```python
from build123d import *

# Parameters (mm, degrees)
BOSS_EXTRUDE1_DEPTH      = 6.35
BOSS_EXTRUDE1_DEPTH_BACK = 6.35
SKETCH2_R                = 25.4
SHELL1_T                 = -2
BOSS_EXTRUDE2_DEPTH      = 6.35
BOSS_EXTRUDE2_DEPTH_BACK = 6.35
CUT_EXTRUDE1_DEPTH       = 44.444866103
SKETCH10_W               = 3.18
SKETCH10_H               = 12.7
CUT_EXTRUDE2_DEPTH       = 44.444866103
FILLET1_R                = 3.175
CUT_EXTRUDE4_REACH       = 63.003
SKETCH11_W               = 12.7
SKETCH11_H               = 3.18
FILLET2_R                = 1.5875
FILL_START               = -6.35
FILL_PATTERN1_OUTLINE_R  = 1.190625
FILL_PATTERN1_DEPTH      = 2


# Read off the part's stored shape, not the designer's step: Fill Pattern1
with BuildPart() as part:
    # Sketch2 → Boss-Extrude1 (new, two sides: drawn at the far end of the back side and taken through both)
    with BuildSketch(Plane(origin=(0, 0, 0), x_dir=(1, 0, 0), z_dir=(0, 1, 0)).offset(-BOSS_EXTRUDE1_DEPTH_BACK)):
        with Locations(Location((0, 0, 0), (0, 0, 270))):
            Circle(SKETCH2_R)
    extrude(amount=BOSS_EXTRUDE1_DEPTH + BOSS_EXTRUDE1_DEPTH_BACK)

    # Shell1
    shell1_openings = [part.faces().sort_by_distance(p)[0] for p in [
        (0, 6.35, 0),
    ]]
    offset(amount=SHELL1_T, openings=shell1_openings, kind=Kind.INTERSECTION)

    # Sketch7 → Boss-Extrude2 (add, two sides: drawn at the far end of the back side and taken through both)
    with BuildSketch(Plane(origin=(0, 0, 0), x_dir=(1, 0, 0), z_dir=(0, 1, 0)).offset(-BOSS_EXTRUDE2_DEPTH_BACK)):
        with BuildLine():
            Line((23.348661632, 10), (32.878661632, 10))
            Line((32.878661632, 10), (32.878661632, -10))
            Line((32.878661632, -10), (23.348661632, -10))
            ThreePointArc((23.348661632, -10), (25.4, 0), (23.348661632, 10))
        make_face()
    extrude(amount=BOSS_EXTRUDE2_DEPTH + BOSS_EXTRUDE2_DEPTH_BACK)

    # Sketch9 → Cut-Extrude1 (cut, through all)
    with BuildSketch(Plane(origin=(0, 6.35, 0), x_dir=(1, 0, 0), z_dir=(0, 1, 0))):
        with BuildLine():
            Line((26.003661632, 7.5), (27.053661632, 7.5))
            ThreePointArc((27.053661632, 7.5), (27.760768413, 7.207106781), (28.053661632, 6.5))
            Line((28.053661632, 6.5), (28.053661632, -6.5))
            ThreePointArc((28.053661632, -6.5), (27.760768413, -7.207106781), (27.053661632, -7.5))
            Line((27.053661632, -7.5), (26.003661632, -7.5))
            ThreePointArc((26.003661632, -7.5), (25.296554851, -7.207106781), (25.003661632, -6.5))
            Line((25.003661632, -6.5), (25.003661632, 6.5))
            ThreePointArc((25.003661632, 6.5), (25.296554851, 7.207106781), (26.003661632, 7.5))
        make_face()
    extrude(amount=-CUT_EXTRUDE1_DEPTH, mode=Mode.SUBTRACT)

    # Sketch10 → Cut-Extrude2 (cut, through all)
    with BuildSketch(Plane(origin=(0, 6.35, 0), x_dir=(1, 0, 0), z_dir=(0, 1, 0))):
        with Locations((31.288661632, 0)):
            Rectangle(SKETCH10_W, SKETCH10_H)
    extrude(amount=-CUT_EXTRUDE2_DEPTH, mode=Mode.SUBTRACT)

    # Fillet1
    fillet1_edges = [part.edges().sort_by_distance(p)[0] for p in [
        (23.348661632, 0, 10),
        (23.348661632, 0, -10),
        (32.878661632, 0, -10),
        (32.878661632, 0, 10),
    ]]
    fillet(fillet1_edges, radius=FILLET1_R)

    # Sketch11 → Cut-Extrude4 (cut, up to next)
    with BuildSketch(Plane(origin=(29.698661632, 0, 0), x_dir=(0, 0, -1), z_dir=(1, 0, 0)), mode=Mode.PRIVATE) as cut_extrude4_sk1:
        with Locations((0, -4.76)):
            Rectangle(SKETCH11_W, SKETCH11_H)
    cut_extrude4_tool1 = extrude(cut_extrude4_sk1.sketch, amount=-CUT_EXTRUDE4_REACH, mode=Mode.PRIVATE) & part.part
    add(cut_extrude4_tool1.solids().sort_by_distance((29.698662, -4.76, 0))[0], mode=Mode.SUBTRACT)

    # Fillet2
    fillet2_edges = [part.edges().sort_by_distance(p)[0] for p in [
        (29.698661632, 1.59, -6.35),
        (29.698661632, 1.59, 6.35),
    ]]
    fillet(fillet2_edges, radius=FILLET2_R)

    # Fill Pattern1 outline → Fill Pattern1 (cut)
    with BuildSketch(Plane(origin=(0, 0, 0), x_dir=(1, 0, 0), z_dir=(0, 1, 0)).offset(FILL_START)):
        with Locations((0, -19.999996628)):
            Circle(FILL_PATTERN1_OUTLINE_R)
        with Locations((4.330127019, -12.499996628)):
            Circle(FILL_PATTERN1_OUTLINE_R)
        with Locations((4.330127019, -7.499996628)):
            Circle(FILL_PATTERN1_OUTLINE_R)
        with Locations((8.660254038, -4.999996628)):
            Circle(FILL_PATTERN1_OUTLINE_R)
        with Locations((8.660254038, 3.372e-06)):
            Circle(FILL_PATTERN1_OUTLINE_R)
        with Locations((12.990381057, 2.500003372)):
            Circle(FILL_PATTERN1_OUTLINE_R)
        with Locations((12.990381057, 7.500003372)):
            Circle(FILL_PATTERN1_OUTLINE_R)
        with Locations((8.660254038, 15.000003372)):
            Circle(FILL_PATTERN1_OUTLINE_R)
        with Locations((-12.990381057, -12.499996628)):
            Circle(FILL_PATTERN1_OUTLINE_R)
        with Locations((-4.330127019, -12.499996628)):
            Circle(FILL_PATTERN1_OUTLINE_R)
        with Locations((0, -9.999996628)):
            Circle(FILL_PATTERN1_OUTLINE_R)
        with Locations((0, -4.999996628)):
            Circle(FILL_PATTERN1_OUTLINE_R)
        with Locations((4.330127019, -2.499996628)):
            Circle(FILL_PATTERN1_OUTLINE_R)
        with Locations((4.330127019, 2.500003372)):
            Circle(FILL_PATTERN1_OUTLINE_R)
        with Locations((8.660254038, 5.000003372)):
            Circle(FILL_PATTERN1_OUTLINE_R)
        with Locations((8.660254038, 10.000003372)):
            Circle(FILL_PATTERN1_OUTLINE_R)
        with Locations((17.320508076, 10.000003372)):
            Circle(FILL_PATTERN1_OUTLINE_R)
        with Locations((-4.330127019, -17.499996628)):
            Circle(FILL_PATTERN1_OUTLINE_R)
        with Locations((4.330127019, -17.499996628)):
            Circle(FILL_PATTERN1_OUTLINE_R)
        with Locations((8.660254038, -14.999996628)):
            Circle(FILL_PATTERN1_OUTLINE_R)
        with Locations((17.320508076, -4.999996628)):
            Circle(FILL_PATTERN1_OUTLINE_R)
        with Locations((17.320508076, -9.999996628)):
            Circle(FILL_PATTERN1_OUTLINE_R)
        with Locations((12.990381057, -12.499996628)):
            Circle(FILL_PATTERN1_OUTLINE_R)
        with Locations((0, -14.999996628)):
            Circle(FILL_PATTERN1_OUTLINE_R)
        with Locations((-8.660254038, -14.999996628)):
            Circle(FILL_PATTERN1_OUTLINE_R)
        with Locations((12.990381057, 12.500003372)):
            Circle(FILL_PATTERN1_OUTLINE_R)
        with Locations((17.320508076, 5.000003372)):
            Circle(FILL_PATTERN1_OUTLINE_R)
        with Locations((17.320508076, 3.372e-06)):
            Circle(FILL_PATTERN1_OUTLINE_R)
        with Locations((12.990381057, -2.499996628)):
            Circle(FILL_PATTERN1_OUTLINE_R)
        with Locations((12.990381057, -7.499996628)):
            Circle(FILL_PATTERN1_OUTLINE_R)
        with Locations((8.660254038, -9.999996628)):
            Circle(FILL_PATTERN1_OUTLINE_R)
        with Locations((-8.660254038, 10.000003372)):
            Circle(FILL_PATTERN1_OUTLINE_R)
        with Locations((-8.660254038, 5.000003372)):
            Circle(FILL_PATTERN1_OUTLINE_R)
        with Locations((-12.990381057, 2.500003372)):
            Circle(FILL_PATTERN1_OUTLINE_R)
        with Locations((-12.990381057, -2.499996628)):
            Circle(FILL_PATTERN1_OUTLINE_R)
        with Locations((0, 10.000003372)):
            Circle(FILL_PATTERN1_OUTLINE_R)
        with Locations((0, 15.000003372)):
            Circle(FILL_PATTERN1_OUTLINE_R)
        with Locations((-17.320508076, -4.999996628)):
            Circle(FILL_PATTERN1_OUTLINE_R)
        with Locations((-12.990381057, 7.500003372)):
            Circle(FILL_PATTERN1_OUTLINE_R)
        with Locations((-12.990381057, 12.500003372)):
            Circle(FILL_PATTERN1_OUTLINE_R)
        with Locations((-8.660254038, 15.000003372)):
            Circle(FILL_PATTERN1_OUTLINE_R)
        with Locations((-17.320508076, 10.000003372)):
            Circle(FILL_PATTERN1_OUTLINE_R)
        with Locations((-17.320508076, 5.000003372)):
            Circle(FILL_PATTERN1_OUTLINE_R)
        with Locations((-17.320508076, 3.372e-06)):
            Circle(FILL_PATTERN1_OUTLINE_R)
        with Locations((-4.330127019, 17.500003372)):
            Circle(FILL_PATTERN1_OUTLINE_R)
        with Locations((-4.330127019, 12.500003372)):
            Circle(FILL_PATTERN1_OUTLINE_R)
        with Locations((0, 5.000003372)):
            Circle(FILL_PATTERN1_OUTLINE_R)
        with Locations((0, 3.372e-06)):
            Circle(FILL_PATTERN1_OUTLINE_R)
        with Locations((-4.330127019, -2.499996628)):
            Circle(FILL_PATTERN1_OUTLINE_R)
        with Locations((-4.330127019, -7.499996628)):
            Circle(FILL_PATTERN1_OUTLINE_R)
        with Locations((-8.660254038, -9.999996628)):
            Circle(FILL_PATTERN1_OUTLINE_R)
        with Locations((-17.320508076, -9.999996628)):
            Circle(FILL_PATTERN1_OUTLINE_R)
        with Locations((4.330127019, 17.500003372)):
            Circle(FILL_PATTERN1_OUTLINE_R)
        with Locations((-4.330127019, 7.500003372)):
            Circle(FILL_PATTERN1_OUTLINE_R)
        with Locations((-4.330127019, 2.500003372)):
            Circle(FILL_PATTERN1_OUTLINE_R)
        with Locations((-8.660254038, 3.372e-06)):
            Circle(FILL_PATTERN1_OUTLINE_R)
        with Locations((-8.660254038, -4.999996628)):
            Circle(FILL_PATTERN1_OUTLINE_R)
        with Locations((-12.990381057, -7.499996628)):
            Circle(FILL_PATTERN1_OUTLINE_R)
        with Locations((0, 20.000003372)):
            Circle(FILL_PATTERN1_OUTLINE_R)
        with Locations((4.330127019, 12.500003372)):
            Circle(FILL_PATTERN1_OUTLINE_R)
        with Locations((4.330127019, 7.500003372)):
            Circle(FILL_PATTERN1_OUTLINE_R)
    extrude(amount=FILL_PATTERN1_DEPTH, mode=Mode.SUBTRACT)


solid = part.part
```
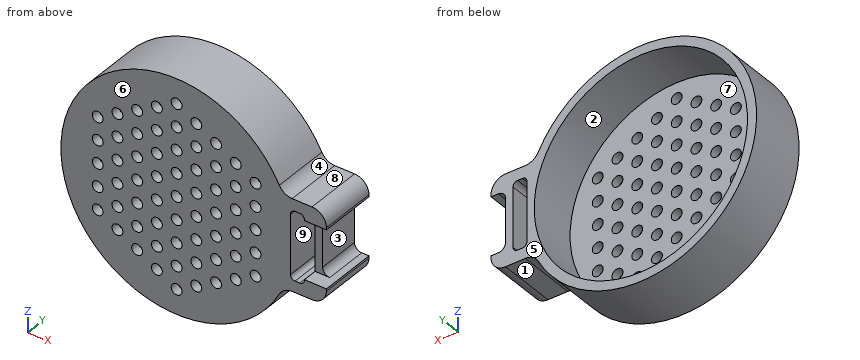
For this review, take the finished solid that the model builds, in its own axes (mm). Face numbers are marked on the shaded views. A direction names the side the tool comes from. Round coordinates to 2 decimals unless told otherwise and drop trailing zeros. Use one line per item in the form item = value.
Q1. Consider section A-A (y = 4). State how many separate pieces and enclosed holes the cut face has, then the cut area to 3 significant figures.
Resolved:
separate_pieces = 1
enclosed_holes = 2
area = 382 mm²
Q2. To check wall thickness, follow probe 1 along Z at (x, y) = (26.5, 4.25); probe 2 along Z at (x, y) = (0.5, -4.25); probe 3 along X at (y, z) = (-5.5, -18). State the ranges of each line that lie inside material, in increasing order. Write a range as from..to.
Resolved:
probe_1 = -10..-7.5, 7.5..10
probe_2 = -25.4..-23.39, 23.39..25.4
probe_3 = -17.92..-5.41, -3.25..3.25, 5.41..17.92
Q3. Machinability: for the marked faces 5, 6, 7, 8 and 9, which of the approach directions +Z, -Z, +X, -X, +Y, -Y give a long, thin tool a straight path to every point of the face, cutting with its end or side? Answer none if there is none.
Resolved:
face_5 = +Z, -Z, +X, -X, +Y
face_6 = +Z, -Z, +X, -X, -Y
face_7 = +Y
face_8 = +Z, +X, +Y, -Y
face_9 = +Y, -Y
Q4. The part is to be moulded in two halves that separate along Z. For the marked faces 1, 2, 3 and 4, say which applies: released by +Z, released by -Z, zero draft, split by the parting line, or undercut.
Resolved:
face_1 = released by -Z
face_2 = undercut
face_3 = undercut
face_4 = released by +Z
Q5. Clearance check with flat-ended pins moving along their axes: pin 1 Ø6 at (x, y) = (13.5, 4) entering from -Z; pin 2 Ø2.5 at (x, z) = (-8.66, 15) entering from +Y; pin 3 Ø2.5 at (x, z) = (8.66, 10) entering from -Y. State where each tip first meets the part, or that it passes through.
Resolved:
pin_1 = -23.13
pin_2 = -4.35
pin_3 = -6.35
